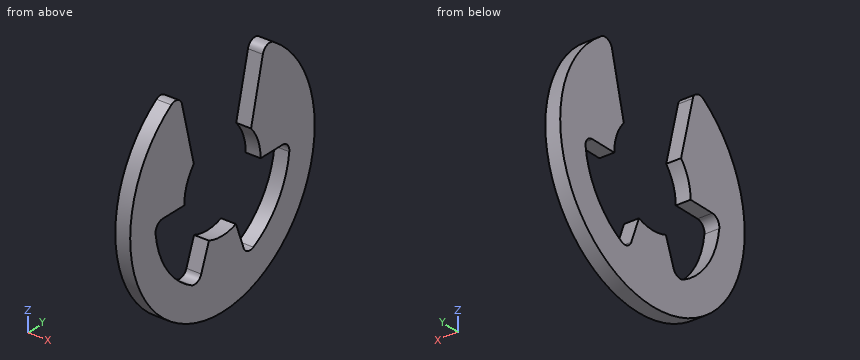
from build123d import *

# Parameters (mm, degrees)
EXTRUDE1_DEPTH = 0.5
FILLET1_R      = 0.6


with BuildPart() as part:
    # Sketch1 → Extrude1 (new body, symmetric)
    with BuildSketch(Plane(origin=(0, 0, 0), x_dir=(0, 0, -1), z_dir=(1, 0, 0))):
        with BuildLine():
            Line((-6.981705618, -3.642994877), (-2.156287319, -2.445))
            ThreePointArc((-2.156287319, -2.445), (-1.152584053, -3.04945077), (0, -3.26))
            Line((0, -3.26), (0, -5.747096774))
            ThreePointArc((0, -5.747096774), (3.267381482, -4.727931851), (5.375916774, -2.031905551))
            Line((5.375916774, -2.031905551), (3.04945077, -1.152584053))
            ThreePointArc((3.04945077, -1.152584053), (3.26, 0), (3.04945077, 1.152584053))
            Line((3.04945077, 1.152584053), (5.375916774, 2.031905551))
            ThreePointArc((5.375916774, 2.031905551), (3.267381482, 4.727931851), (0, 5.747096774))
            Line((0, 5.747096774), (0, 3.26))
            ThreePointArc((0, 3.26), (-1.152584053, 3.04945077), (-2.156287319, 2.445))
            Line((-2.156287319, 2.445), (-6.981705618, 3.642994877))
            ThreePointArc((-6.981705618, 3.642994877), (7.875, 0), (-6.981705618, -3.642994877))
        make_face()
    extrude(amount=EXTRUDE1_DEPTH, both=True)

    # Fillet1
    fillet1_edges = [part.edges().sort_by_distance(p)[0] for p in [
        (0, -3.642994877, 6.981705618),
        (0, -5.747096774, 0),
        (0, -2.031905551, -5.375916774),
        (0, 2.031905551, -5.375916774),
        (0, 5.747096774, 0),
        (0, 3.642994877, 6.981705618),
    ]]
    fillet(fillet1_edges, radius=FILLET1_R)


solid = part.part
The listing builds one solid part. Answer for the finished solid, in the listing's coordinates (mm). Round coordinates to 2 decimals unless told otherwise and drop trailing zeros. Write each loop counter-clockwise with the first axis right and the second up, starting at its lowest first coordinate (ties: lowest second). Pieces come first, ordered by that corner, then holes. Notation, with made-up numbers: M 89,66.5 L 104,66.5 A29 ccw 104,105.5 Z; hole C 27,-2.75 d10. An arc over 180 degrees is marked long. Write each question's results on one line, items separated by ' | '. Start each with the question number.
Item 1: A cutting plane is placed at B-B on z = -1.5. Write down the section's boundary in (x, y), and give its area (3 significant figures).
Item 2: Straight lines are drawn through the part: L1, parallel to Y at x = 0.3, z = -3.5; L2, parallel to Y at x = -0.1, z = -4.75; L3, parallel to Y at x = -0.3, z = 3. For each, find the intervals that lie inside material, in ascending order. Write a range as [from, to].
Item 3: A cutting plane is placed at A-A on x = -0.05. Write down the section's boundary in (y, z) (3 decimals).
Item 4: A cutting plane is placed at C-C on y = 3. Write down the section's boundary in (x, z).
Item 5: Flat-ended cylindrical pins translate along their axes: pin 1 Ø1.5 at (y, z) = (1, -1.5) entering from -X; pin 2 Ø0.5 at (x, y) = (0, -4) entering from -Z. Find the tip coordinate at first contact, or state that the pin passes through.
Item 6: A cutting plane is placed at D-D on y = 0. Write down the section's boundary in (x, z) (3 decimals), and give its area (4 significant figures).
Check sheet entries:
1) outline: M -0.5,-7.73 L 0.5,-7.73 L 0.5,-5.55 L -0.5,-5.55 Z; M -0.5,5.55 L 0.5,5.55 L 0.5,7.73 L -0.5,7.73 Z | area: 4.37 mm²
2) L1: [-7.05, -4.56], [-1.32, 1.32], [4.56, 7.05] | L2: [-6.28, -3.24], [-1.8, 1.8], [3.24, 6.28] | L3: [-7.28, -2.65], [2.65, 7.28]
3) outline: M -5.708,-0.67 A0.6 cw -5.112,0 L -3.26,0 A3.26 cw -2.445,2.156 L -3.449,6.2 A0.6 ccw -4.364,6.555 A7.875 ccw long 4.364,6.555 A0.6 ccw 3.449,6.2 L 2.445,2.156 A3.26 cw 3.26,0 L 5.112,0 A0.6 cw 5.708,-0.67 A5.747 cw 2.645,-5.102 A0.6 cw 1.807,-4.782 L 1.153,-3.049 A3.26 cw -1.153,-3.049 L -1.807,-4.782 A0.6 cw -2.645,-5.102 A5.747 cw Z
4) outline: M -0.5,-7.28 L 0.5,-7.28 L 0.5,-4.9 L -0.5,-4.9 Z; M -0.5,1.28 L 0.5,1.28 L 0.5,4.39 L -0.5,4.39 Z
5) pin 1: through | pin 2: z = -6.92
6) outline: M -0.5,-7.875 L 0.5,-7.875 L 0.5,-3.26 L -0.5,-3.26 Z | area: 4.615 mm²
